from build123d import *

# Parameters (mm, degrees)
SKETCH1_R           = 127.5
SKETCH1_R_2         = 80
SKETCH1_R_3         = 6
BOSS_EXTRUDE1_DEPTH = 8
SKETCH2_R           = 84
SKETCH2_R_2         = 80
BOSS_EXTRUDE2_DEPTH = 525.2
SKETCH3_R           = 84
SKETCH3_R_2         = 80
SKETCH5_R           = 84
SKETCH5_R_2         = 80
BOSS_EXTRUDE3_DEPTH = 1325.9


with BuildPart() as part:
    # Sketch1 → Boss-Extrude1 (new body)
    with BuildSketch(Plane(origin=(0, 0, 0), x_dir=(0, 0, -1), z_dir=(1, 0, 0))):
        Circle(SKETCH1_R)
        Circle(SKETCH1_R_2, mode=Mode.SUBTRACT)
        with Locations((0, 109)):
            Circle(SKETCH1_R_3, mode=Mode.SUBTRACT)
        with Locations((77.074639149, 77.074639149)):
            Circle(SKETCH1_R_3, mode=Mode.SUBTRACT)
        with Locations((109, 0)):
            Circle(SKETCH1_R_3, mode=Mode.SUBTRACT)
        with Locations((77.074639149, -77.074639149)):
            Circle(SKETCH1_R_3, mode=Mode.SUBTRACT)
        with Locations((0, -109)):
            Circle(SKETCH1_R_3, mode=Mode.SUBTRACT)
        with Locations((-77.074639149, -77.074639149)):
            Circle(SKETCH1_R_3, mode=Mode.SUBTRACT)
        with Locations((-109, 0)):
            Circle(SKETCH1_R_3, mode=Mode.SUBTRACT)
        with Locations((-77.074639149, 77.074639149)):
            Circle(SKETCH1_R_3, mode=Mode.SUBTRACT)
    extrude(amount=BOSS_EXTRUDE1_DEPTH)

    # Sketch2 → Boss-Extrude2 (add)
    with BuildSketch(Plane(origin=(8, 0, 0), x_dir=(0, 0, -1), z_dir=(1, 0, 0))):
        Circle(SKETCH2_R)
        Circle(SKETCH2_R_2, mode=Mode.SUBTRACT)
    extrude(amount=BOSS_EXTRUDE2_DEPTH)

    # Sweep1: sweep along a path in Sketch4
    with BuildLine(Plane.XY) as sweep1_path:
        ThreePointArc((533.2, 0), (694.844610179, -66.955389821), (761.8, -228.6))
    # Sketch3 → Sweep1 (sweep)
    with BuildSketch(Plane(origin=(533.2, 0, 0), x_dir=(0, 0, -1), z_dir=(1, 0, 0))):
        Circle(SKETCH3_R)
        Circle(SKETCH3_R_2, mode=Mode.SUBTRACT)
    sweep(path=sweep1_path.line)

    # Sketch5 → Boss-Extrude3 (add)
    with BuildSketch(Plane.XZ.offset(228.6)):
        with Locations((761.8, 0)):
            Circle(SKETCH5_R)
        with Locations((761.8, 0)):
            Circle(SKETCH5_R_2, mode=Mode.SUBTRACT)
    extrude(amount=BOSS_EXTRUDE3_DEPTH)


solid = part.part
Model file for the job. Use its own axes, mm. A direction names the side the tool comes from. Round coordinates to 2 decimals unless told otherwise and drop trailing zeros. Loops run counter-clockwise (first coordinate to the right, second up) from the corner with the lowest first, then second, coordinate; pieces in that order, holes last. Notation, with made-up numbers: M 59,-28 L 95,-28 A5 cw 95,-24 Z; hole C 22.25,-30.75 d6. An arc over 180 degrees is marked long. One line per question, with ' | ' between items.
1) Band-saw the part on C-C (x = 128). Give the cut face in (y, z), then the cut area to 3 significant figures.
Solved:
outline: C 0,0 d168; hole C 0,0 d160 | area: 2,060 mm²
2) Band-saw the part on A-A (z = 36.5). Give the cut face in (x, y), then the cut area to 3 significant figures.
Solved:
outline: M 0,-122.16 L 8,-122.16 L 8,-75.66 L 533.2,-75.66 A152.94 cw 686.14,-228.6 L 686.14,-1554.5 L 690.61,-1554.5 L 690.61,-228.6 A157.41 ccw 533.2,-71.19 L 0,-71.19 Z; M 0,71.19 L 533.2,71.19 A299.79 cw 832.99,-228.6 L 832.99,-1554.5 L 837.46,-1554.5 L 837.46,-228.6 A304.26 ccw 533.2,75.66 L 8,75.66 L 8,122.16 L 0,122.16 Z | area: 20,600 mm²
3) 3-axis set-ups, long thin cutter, end or side, ignore diameter. For faces 5 (the cylindrical face through (262.87, -78.1, 17.34)), 6 (the flat face through (793, -1554.5, -74)), 7 (the cylindrical face through (835.7, -882.27, -30.64)), 8 (the cylindrical face through (266.92, 25.23, -80.12)): which of +Z, -Z, +X, -X, +Y, -Y reach the whole face in a straight line?
Solved:
face 5: -X | face 6: +Z, -Z, +X, -X, -Y | face 7: -Y | face 8: none
4) Mould opens along X. For faces 1 (the flat face through (0, 58.5, -54.9)), 2 (the cylindrical face through (3.94, -124.47, 27.64)), 3 (the flat face through (8, 2, 87)), 4 (the cylindrical face through (839.395, -882.269, -32.172)) say: +X half, -X half, draft (parallel to the pull), parting line (faces both ways), or undercut.
Solved:
face 1: -X half | face 2: draft | face 3: undercut | face 4: parting line
5) Drill centre lines: line 1 along Y through (x, z) = (5, 0); line 2 along Y through (x, z) = (4, -109); line 3 along X through (y, z) = (-127, 10). Where is each one in solid material? Low to high.
Solved:
line 1: y = -127.5 to -115, -103 to -80, 80 to 103, 115 to 127.5 | line 2: y = -66.15 to -6, 6 to 66.15 | line 3: x = 0 to 8, 636.93 to 642.5, 823.93 to 828.2
6) Band-saw the part on B-B (y = -909.5). Give the cut face in (x, z), then the cut area to 3 significant figures.
Solved:
outline: C 761.8,0 d168; hole C 761.8,0 d160 | area: 2,060 mm²
7) Band-saw the part on D-D (z = -35). Give the cut face in (x, y), then the cut area to 3 significant figures.
Solved:
outline: M 0,-122.6 L 8,-122.6 L 8,-76.36 L 533.2,-76.36 A152.24 cw 685.44,-228.6 L 685.44,-1554.5 L 689.86,-1554.5 L 689.86,-228.6 A156.66 ccw 533.2,-71.94 L 0,-71.94 Z; M 0,71.94 L 533.2,71.94 A300.54 cw 833.74,-228.6 L 833.74,-1554.5 L 838.16,-1554.5 L 838.16,-228.6 A304.96 ccw 533.2,76.36 L 8,76.36 L 8,122.6 L 0,122.6 Z | area: 20,400 mm²
8) Flat gauge pins, fed straight in: pin 1 (9.5 mm diameter, centred on y = 0, z = 109, fed in from -X); pin 2 (1.5 mm diameter, centred on x = 175.5, z = 65, fed in from +Y); pin 3 (3 mm diameter, centred on x = 691.5, y = -1036.5, fed in from -Z); pin 4 (6 mm diameter, centred on x = 416, z = 19.5, fed in from +Y). Where does each tip first touch, or does it go through?
Solved:
pin 1: passes through | pin 2: stops at y = 54.11 | pin 3: stops at z = -48.19 | pin 4: stops at y = 82.36
